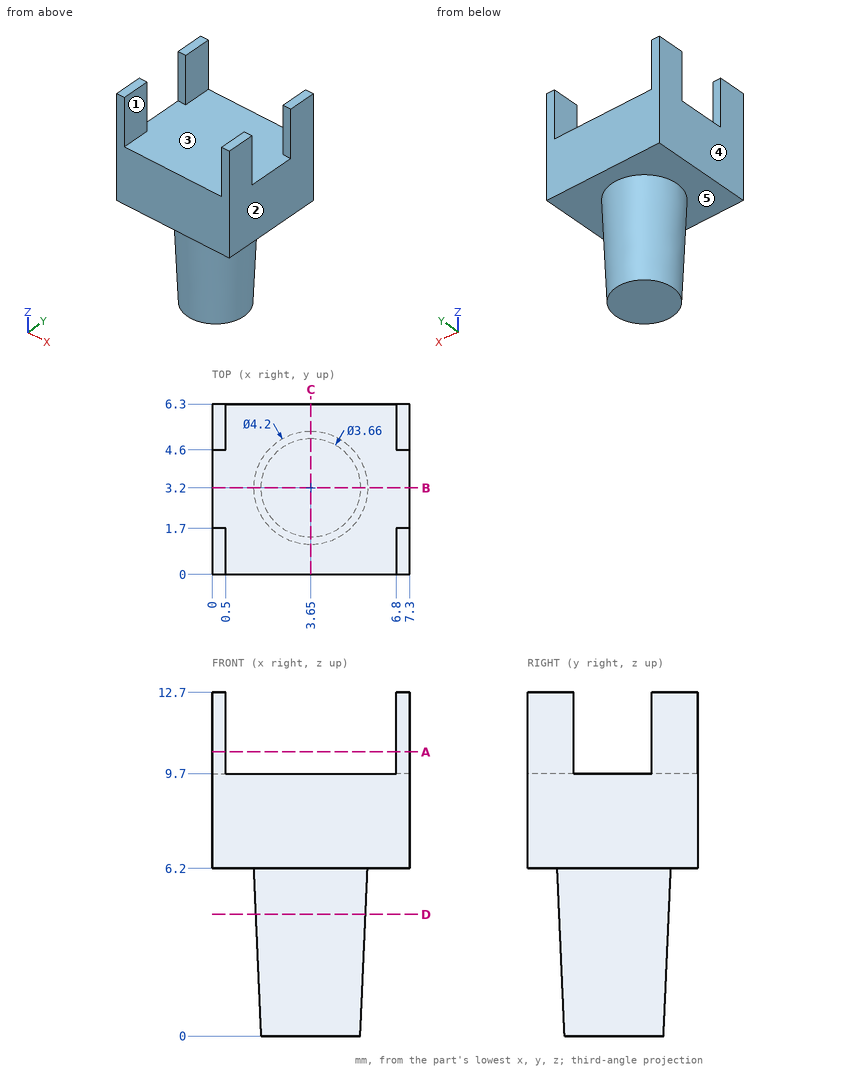
Could you check a few things on this drawing? It's one solid part, dimensions in mm from its lowest x, y, z. A direction names the side the tool comes from. Round coordinates to 2 decimals unless told otherwise and drop trailing zeros. Write each loop counter-clockwise with the first axis right and the second up, starting at its lowest first coordinate (ties: lowest second). Pieces come first, ordered by that corner, then holes. Notation, with made-up numbers: (63.25, 69.5) -> (72.25, 69.5) arc R28 cw to (72.25, 90.5) -> close; hole circle Ø11 at (-29.75, 80.25). An arc over 180 degrees is marked (long way). One line per question, with ' | ' between items. Start each with the question number.
1) Suppose I cut it at D-D on z = 4.5. Write out the boundary of the cut face in (x, y), then the cut area to 3 significant figures.
2) On a 3-axis mill with a long thin cutter (end or side, diameter ignored), from which of +Z, -Z, +X, -X, +Y, -Y can I reach the whole of each face in a straight line? I mean the marked faces 1 and 2. Say none if no direction works.
3) If we mould it in two halves opening along X, with no side actions, what happens to the marked faces 3, 4 and 5? For each: released by +X, released by -X, zero draft, split by the parting line, or undercut.
4) Suppose I cut it at B-B on y = 3.2. Write out the boundary of the cut face in (x, z), then the cut area to 3 significant figures.
5) I'm going to push flat-ended pins straight in: P1, Ø1, axis at y = 1, z = 4, coming from the -X side; P2, Ø1.9, axis at x = 4, y = 4, coming from the +Z side. Where does each tip first touch, or does it pass through?
6) Suppose I cut it at C-C on x = 3.65. Write out the boundary of the cut face in (y, z).
7) I need wall thicknesses on line 1 (Z direction, x = 6, y = 4); line 2 (X direction, y = 5.5, z = 11.75); line 3 (Z direction, x = 4, y = 3.75). Which ranges of each line are inside material? Lowest first, please. Write a range as [from, to].
8) Suppose I cut it at A-A on z = 10.5. Write out the boundary of the cut face in (x, y).
Return value:
1) outline: circle Ø4.05 at (3.65, 3.2) | area: 12.9 mm2
2) face 1: +Z, +Y, -Y | face 2: +Z, -Z, +X, +Y, -Y
3) face 3: undercut | face 4: released by -X | face 5: zero draft
4) outline: (0, 6.2) -> (1.55, 6.2) -> (1.82, 0) -> (5.48, 0) -> (5.75, 6.2) -> (7.3, 6.2) -> (7.3, 9.7) -> (0, 9.7) -> close | area: 49.9 mm2
5) P1: stops at x = 2.59 | P2: stops at z = 9.7
6) outline: (0, 6.2) -> (1.1, 6.2) -> (1.37, 0) -> (5.03, 0) -> (5.3, 6.2) -> (6.3, 6.2) -> (6.3, 9.7) -> (0, 9.7) -> close
7) line 1: z = [6.2, 9.7] | line 2: x = [0, 0.5], [6.8, 7.3] | line 3: z = [0, 9.7]
8) outline: (0, 0) -> (0.5, 0) -> (0.5, 1.7) -> (0, 1.7) -> close; (0, 4.6) -> (0.5, 4.6) -> (0.5, 6.3) -> (0, 6.3) -> close; (6.8, 0) -> (7.3, 0) -> (7.3, 1.7) -> (6.8, 1.7) -> close; (6.8, 4.6) -> (7.3, 4.6) -> (7.3, 6.3) -> (6.8, 6.3) -> close
